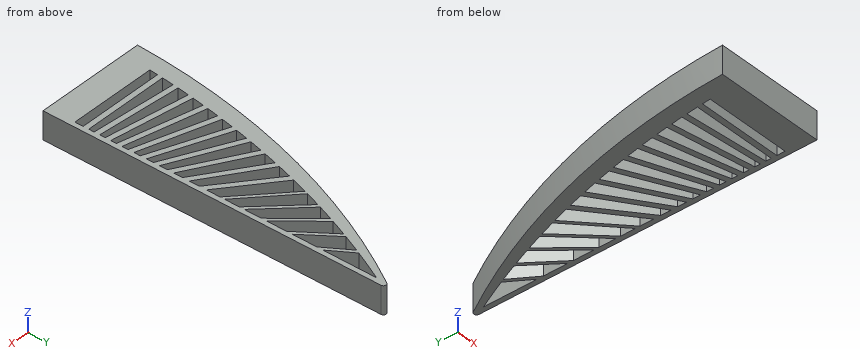
```python
from build123d import *

# Parameters (mm, degrees)
BOSS_EXTRUDE4_DEPTH = 10
BOSS_EXTRUDE5_DEPTH = 10


with BuildPart() as part:
    # Sketch5 → Boss-Extrude4 (new body)
    with BuildSketch(Plane.XY):
        with BuildLine():
            Line((0, 0), (0, 122.364670388))
            ThreePointArc((0, 122.364670388), (-0.722776757, 123.325475922), (-1.846294547, 122.89738564))
            ThreePointArc((-1.846294547, 122.89738564), (-28.906490201, 63.952063235), (-39.720316086, 0))
            Line((-39.720316086, 0), (0, 0))
        make_face()
        with BuildLine():
            Line((-1.8, 10), (-33.298, 10))
            ThreePointArc((-33.298, 10), (-22.875707389, 66.135343677), (-1.8, 119.197717832))
            Line((-1.8, 119.197717832), (-1.8, 10))
        make_face(mode=Mode.SUBTRACT)
    extrude(amount=BOSS_EXTRUDE4_DEPTH)

    # Sketch8 → Boss-Extrude5 (add)
    with BuildSketch(Plane.XY):
        with BuildLine():
            Line((-33.02290127, 13), (-1.8, 13))
            Line((-1.8, 13), (-1.8, 15))
            Line((-1.8, 15), (-32.822260718, 15))
            ThreePointArc((-32.822260718, 15), (-32.924290216, 14.00017147), (-33.02290127, 13))
        make_face()
        with BuildLine():
            Line((-31.551287828, 25.428873475), (-1.8, 20.944756944))
            Line((-1.8, 20.944756944), (-1.8, 22.967345922))
            Line((-1.8, 22.967345922), (-31.267160482, 27.408638756))
            ThreePointArc((-31.267160482, 27.408638756), (-31.410907676, 26.418997727), (-31.551287828, 25.428873475))
        make_face()
        with BuildLine():
            Line((-32.351201095, 19.239482352), (-1.8, 16.950071453))
            Line((-1.8, 16.950071453), (-1.8, 18.955679124))
            Line((-1.8, 18.955679124), (-32.108897466, 21.226932551))
            ThreePointArc((-32.108897466, 21.226932551), (-32.231741124, 20.233413716), (-32.351201095, 19.239482352))
        make_face()
        with BuildLine():
            Line((-30.618838123, 31.608168854), (-1.8, 25.030709106))
            Line((-1.8, 25.030709106), (-1.8, 27.082138941))
            Line((-1.8, 27.082138941), (-30.292091958, 33.585023866))
            ThreePointArc((-30.292091958, 33.585023866), (-30.457149134, 32.596874717), (-30.618838123, 31.608168854))
        make_face()
        with BuildLine():
            Line((-29.545931615, 37.81700869), (-1.8, 29.258858956))
            Line((-1.8, 29.258858956), (-1.8, 31.351837274))
            Line((-1.8, 31.351837274), (-29.175137635, 39.795616712))
            ThreePointArc((-29.175137635, 39.795616712), (-29.3622281, 38.806630061), (-29.545931615, 37.81700869))
        make_face()
        with BuildLine():
            Line((-28.320844309, 44.095333315), (-1.8, 33.687092884))
            Line((-1.8, 33.687092884), (-1.8, 35.835600273))
            Line((-1.8, 35.835600273), (-27.903926427, 46.080219158))
            ThreePointArc((-27.903926427, 46.080219158), (-28.114096999, 45.088135758), (-28.320844309, 44.095333315))
        make_face()
        with BuildLine():
            Line((-26.927669735, 50.484015361), (-1.8, 38.383681924))
            Line((-1.8, 38.383681924), (-1.8, 40.603496684))
            Line((-1.8, 40.603496684), (-26.461878817, 52.479526575))
            ThreePointArc((-26.461878817, 52.479526575), (-26.696512847, 51.482176784), (-26.927669735, 50.484015361))
        make_face()
        with BuildLine():
            Line((-25.34575305, 57.025462495), (-1.8, 43.431924442))
            Line((-1.8, 43.431924442), (-1.8, 45.741299663))
            Line((-1.8, 45.741299663), (-24.827629625, 59.035712413))
            ThreePointArc((-24.827629625, 59.035712413), (-25.088465651, 58.031044767), (-25.34575305, 57.025462495))
        make_face()
        with BuildLine():
            Line((-23.548915199, 63.764175049), (-1.8, 48.936721808))
            Line((-1.8, 48.936721808), (-1.8, 51.357293007))
            Line((-1.8, 51.357293007), (-22.974243013, 65.792960042))
            ThreePointArc((-22.974243013, 65.792960042), (-23.26339795, 64.77908275), (-23.548915199, 63.764175049))
        make_face()
        with BuildLine():
            Line((-21.504437213, 70.747227787), (-1.8, 55.034267194))
            Line((-1.8, 55.034267194), (-1.8, 57.592312347))
            Line((-1.8, 57.592312347), (-20.868191149, 72.797909588))
            ThreePointArc((-20.868191149, 72.797909588), (-21.188186233, 71.773149512), (-21.504437213, 70.747227787))
        make_face()
        with BuildLine():
            Line((-19.009701273, 78.507124213), (-1.8, 62.539493808))
            Line((-1.8, 62.539493808), (-1.8, 64.176455444))
            Line((-1.8, 64.176455444), (-18.587222465, 79.752098484))
            ThreePointArc((-18.587222465, 79.752098484), (-18.799157777, 79.129847503), (-19.009701273, 78.507124213))
        make_face()
        with BuildLine():
            Line((-16.685267787, 85.144051641), (-1.8, 69.502691427))
            Line((-1.8, 69.502691427), (-1.8, 71.243382102))
            Line((-1.8, 71.243382102), (-16.22487287, 86.400961786))
            ThreePointArc((-16.22487287, 86.400961786), (-16.455785666, 85.772768735), (-16.685267787, 85.144051641))
        make_face()
        with BuildLine():
            Line((-14.072204317, 92.056761761), (-1.8, 77.440823569))
            Line((-1.8, 77.440823569), (-1.8, 79.306980252))
            Line((-1.8, 79.306980252), (-13.570797112, 93.325752969))
            ThreePointArc((-13.570797112, 93.325752969), (-13.822236892, 92.691548245), (-14.072204317, 92.056761761))
        make_face()
        with BuildLine():
            Line((-11.127713878, 99.276715969), (-1.8, 86.650543681))
            Line((-1.8, 86.650543681), (-1.8, 88.670070899))
            Line((-1.8, 88.670070899), (-10.581907863, 100.557429702))
            ThreePointArc((-10.581907863, 100.557429702), (-10.855568937, 99.917395903), (-11.127713878, 99.276715969))
        make_face()
        with BuildLine():
            Line((-7.801640698, 106.835271915), (-1.8, 97.555550659))
            Line((-1.8, 97.555550659), (-1.8, 99.765221681))
            Line((-1.8, 99.765221681), (-7.207784689, 108.126724319))
            ThreePointArc((-7.207784689, 108.126724319), (-7.505493193, 107.481357019), (-7.801640698, 106.835271915))
        make_face()
    extrude(amount=BOSS_EXTRUDE5_DEPTH)


solid = part.part
```
Work out the finished part from the listing and answer in its coordinate system (mm). Coordinates: 2 decimals unless noted, no trailing zeros. Loops run counter-clockwise (first coordinate to the right, second up) from the corner with the lowest first, then second, coordinate; pieces in that order, holes last.
1) Section B-B (z = 5.75) is taken. Give the number of separate pieces and of enclosed holes in the cut face, plus the area to 3 significant figures.
Results:
separate pieces: 1
enclosed holes: 16
area: 1,820 mm2
2) Consider probe 1 along X at (y, z) = (52, 4); probe 2 along X at (y, z) = (103.5, 1.75); probe 3 along X at (y, z) = (87, 1.75). Determine where each line is inside the solid, lowest interval first.
Results:
probe 1: x = -32.26 to -25.47, -16.64 to -12.64, -6.29 to -2.74, -1.8 to 0
probe 2: x = -12.87 to -9.3, -5.64 to -4.22, -1.8 to 0
probe 3: x = -20.53 to -16, -9.83 to -8.26, -2.06 to 0
3) Flat-ended cylindrical pins translate along their axes: pin 1 (5 mm diameter, centred on y = 105.5, z = 5, fed in from -X); pin 2 (1.7 mm diameter, centred on y = 28, z = 4, fed in from -X); pin 3 (2 mm diameter, centred on y = 16, z = 6.5, fed in from -X); pin 4 (3 mm diameter, centred on x = -10.5, y = 68, fed in from -Z). Find the tip coordinate at first contact, or state that the pin passes through.
Results:
pin 1: stops at x = -13.12
pin 2: stops at x = -37.24
pin 3: stops at x = -38.72
pin 4: passes through
4) Section A-A (y = 96) is taken. Give the vertices of the cut face in (x, z), plus the area to 3 significant figures.
Results:
outline: (-16.53, 0) - (-12.49, 0) - (-12.49, 10) - (-16.53, 10) - close; (-8.71, 0) - (-7.22, 0) - (-7.22, 10) - (-8.71, 10) - close; (-1.8, 0) - (0, 0) - (0, 10) - (-1.8, 10) - close
area: 73.4 mm2
